Model file for the job. Use its own axes, mm. A direction names the side the tool comes from. Coordinates: 2 decimals unless noted, no trailing zeros. Write each loop counter-clockwise with the first axis right and the second up, starting at its lowest first coordinate (ties: lowest second). Pieces come first, ordered by that corner, then holes.
Q1. Band-saw the part on D-D, the plane y = -48.5. Write the cut outline in (x, z), plus the area to 3 significant figures.
Q2. Band-saw the part on C-C, the plane y = -26. Write the cut outline in (x, z).
Q3. Which spindle directions (+Z, -Z, +X, -X, +Y, -Y) get a long thin tool onto all of the face, cutting with end or side? Do faces 1 (the flat face through (18, 26.5, 17)), 2 (the flat face through (17.71, -15.74, 43.2)), 3 (the flat face through (-17.063, -2.368, 24.694)). Say none if no direction does.
Q4. Band-saw the part on A-A, the plane x = -51.5. Write the cut outline in (y, z).
Q5. Pin check, flat tips, straight feed: P1, Ø7, axis at x = -51.5, y = 48.5, coming from the +Z side; P2, Ø9.5, axis at y = -27.5, z = 33, coming from the -X side; P3, Ø5, axis at x = 7.5, z = 26.5, coming from the -Y side. Stop position of each tip, or through.
Q6. Band-saw the part on B-B, the plane y = 48.5. Write the cut outline in (x, z), plus the area to 3 significant figures.
Q7. Drill centre lines: probe 1 along Y at (x, z) = (-51.5, 17.25); probe 2 along Y at (x, z) = (51.5, 16.4); probe 3 along X at (y, z) = (48, 17). Where is each one in solid material? Low to high.
Q8. Pull direction Y, two halves, no side cores. Call faces 4 (the flat face through (-56.5, -1, 17)), 5 (the flat face through (-1, 53.5, 17)), 6 (the flat face through (-14.972, -17.284, 37.298)): released by +Y, released by -Y, zero draft, split by the parting line, or undercut.
from build123d import *

# Parameters (mm, degrees)
SKETCH1_W           = 113
SKETCH1_H           = 107
BOSS_EXTRUDE1_DEPTH = 20
SKETCH2_W           = 93
SKETCH2_H           = 87
CUT_EXTRUDE1_DEPTH  = 15
BOSS_EXTRUDE4_DEPTH = 20.5
SKETCH7_W           = 23
SKETCH7_H           = 10
CUT_EXTRUDE2_DEPTH  = 41
SKETCH10_R          = 3.727648652
SKETCH10_R_2        = 3.099940234
SKETCH10_R_3        = 3.503081025
SKETCH10_R_4        = 3.946186921
CUT_EXTRUDE3_DEPTH  = 94.259123843
SKETCH12_R          = 2
CUT_EXTRUDE5_DEPTH  = 10
CUT_EXTRUDE6_DEPTH  = 1.675
SKETCH15_W          = 118.362800564
SKETCH15_H          = 111.14113597
CUT_EXTRUDE7_DEPTH  = 86.907098164


with BuildPart() as part:
    # Sketch1 → Boss-Extrude1 (new body)
    with BuildSketch(Plane.XY):
        Rectangle(SKETCH1_W, SKETCH1_H)
    extrude(amount=BOSS_EXTRUDE1_DEPTH)

    # Sketch2 → Cut-Extrude1 (cut)
    with BuildSketch(Plane(origin=(0, 0, 0), x_dir=(-1, 0, 0), z_dir=(0, 0, -1))):
        Rectangle(SKETCH2_W, SKETCH2_H)
    extrude(amount=-CUT_EXTRUDE1_DEPTH, mode=Mode.SUBTRACT)

    # Sketch9 → Boss-Extrude4 (add, symmetric)
    with BuildSketch(Plane.ZY):
        Polygon((20, -53.5), (51.407822168, -16.069615096), (20, 10.284676901), align=None)
    extrude(amount=BOSS_EXTRUDE4_DEPTH, both=True)

    # Sketch7 → Cut-Extrude2 (cut)
    with BuildSketch(Plane(origin=(0, 0, 15), x_dir=(-1, 0, 0), z_dir=(0, 0, -1))):
        with Locations((-18, 31.5)):
            Rectangle(SKETCH7_W, SKETCH7_H)
        with Locations((14, 31.5)):
            Rectangle(SKETCH7_W, SKETCH7_H)
    extrude(amount=-CUT_EXTRUDE2_DEPTH, mode=Mode.SUBTRACT)

    # Sketch10 → Cut-Extrude3 (cut, through all)
    with BuildSketch(Plane(origin=(0, 0, 0), x_dir=(-1, 0, 0), z_dir=(0, 0, -1))):
        with Locations((-51.5, 48.5)):
            Circle(SKETCH10_R)
        with Locations((51.5, 48.5)):
            Circle(SKETCH10_R_2)
        with Locations((51.5, -48.5)):
            Circle(SKETCH10_R_3)
        with Locations((-51.5, -48.5)):
            Circle(SKETCH10_R_4)
    extrude(amount=-CUT_EXTRUDE3_DEPTH, mode=Mode.SUBTRACT)

    # Sketch12 → Cut-Extrude5 (cut)
    with BuildSketch(Plane(origin=(0, 15.883373682, 13.327732998), x_dir=(1, 0, 0), z_dir=(0, 0.7660444431189817, 0.6427876096865348))):
        with Locations(Location((-15, -19.710025981, 0), (0, 0, 270))):
            Circle(SKETCH12_R)
        with Locations(Location((15, -19.710025981, 0), (0, 0, 270))):
            Circle(SKETCH12_R)
        with Locations(Location((-14.999896364, -39.710025981, 0), (0, 0, 270))):
            Circle(SKETCH12_R)
        with Locations(Location((15, -39.710025981, 0), (0, 0, 270))):
            Circle(SKETCH12_R)
    extrude(amount=-CUT_EXTRUDE5_DEPTH, mode=Mode.SUBTRACT)

    # Sketch14 → Cut-Extrude6 (cut, symmetric)
    with BuildSketch(Plane(origin=(0, 12.053151466, 10.11379495), x_dir=(1, 0, 0), z_dir=(0, 0.7660444431189817, 0.6427876096865348))):
        with BuildLine():
            Line((-20.5, -16.210025981), (-20.5, -23.210025981))
            Line((-20.5, -23.210025981), (-15, -23.210025981))
            ThreePointArc((-15, -23.210025981), (-11.5, -19.710025981), (-15, -16.210025981))
            Line((-15, -16.210025981), (-20.5, -16.210025981))
        make_face()
        with BuildLine():
            Line((-20.5, -36.210025981), (-20.5, -43.210025981))
            Line((-20.5, -43.210025981), (-14.999896364, -43.210025981))
            ThreePointArc((-14.999896364, -43.210025981), (-11.499896364, -39.710025981), (-14.999896364, -36.210025981))
            Line((-14.999896364, -36.210025981), (-20.5, -36.210025981))
        make_face()
        with BuildLine():
            Line((20.5, -43.210025981), (20.5, -36.210025981))
            Line((20.5, -36.210025981), (15, -36.210025981))
            ThreePointArc((15, -36.210025981), (11.5, -39.710025981), (15, -43.210025981))
            Line((15, -43.210025981), (20.5, -43.210025981))
        make_face()
        with BuildLine():
            Line((20.5, -23.210025981), (20.5, -16.210025981))
            Line((20.5, -16.210025981), (15, -16.210025981))
            ThreePointArc((15, -16.210025981), (11.5, -19.710025981), (15, -23.210025981))
            Line((15, -23.210025981), (20.5, -23.210025981))
        make_face()
    extrude(amount=CUT_EXTRUDE6_DEPTH, both=True, mode=Mode.SUBTRACT)

    # Sketch15 → Cut-Extrude7 (cut, through all)
    with BuildSketch(Plane(origin=(0, 0, 15), x_dir=(-1, 0, 0), z_dir=(0, 0, -1))):
        Rectangle(SKETCH15_W, SKETCH15_H)
    extrude(amount=CUT_EXTRUDE7_DEPTH, mode=Mode.SUBTRACT)


solid = part.part
Answer sheet:
1. outline: (-56.5, 15) - (-55, 15) - (-55, 20) - (-56.5, 20) - close; (-48, 15) - (47.55, 15) - (47.55, 20) - (20.5, 20) - (20.5, 24.2) - (-20.5, 24.2) - (-20.5, 20) - (-48, 20) - close; (55.45, 15) - (56.5, 15) - (56.5, 20) - (55.45, 20) - close
1. area: 663 mm2
2. outline: (-56.5, 15) - (56.5, 15) - (56.5, 20) - (20.5, 20) - (20.5, 43.08) - (-20.5, 43.08) - (-20.5, 20) - (-56.5, 20) - close
3. face 1: +Z, -Z
3. face 2: +X
3. face 3: -X
4. outline: (-53.5, 15) - (-52, 15) - (-52, 20) - (-53.5, 20) - close; (-45, 15) - (45.4, 15) - (45.4, 20) - (-45, 20) - close; (51.6, 15) - (53.5, 15) - (53.5, 20) - (51.6, 20) - close
5. P1: stops at z = 20
5. P2: stops at x = -20.5
5. P3: stops at y = -48.73
6. outline: (-56.5, 15) - (-54.6, 15) - (-54.6, 20) - (-56.5, 20) - close; (-48.4, 15) - (47.77, 15) - (47.77, 20) - (-48.4, 20) - close; (55.23, 15) - (56.5, 15) - (56.5, 20) - (55.23, 20) - close
6. area: 497 mm2
7. probe 1: y = -53.5 to -52, -45 to 45.4, 51.6 to 53.5
7. probe 2: y = -53.5 to -52.45, -44.55 to 44.77, 52.23 to 53.5
7. probe 3: x = -56.5 to -54.56, -48.44 to 47.81, 55.19 to 56.5
8. face 4: zero draft
8. face 5: released by +Y
8. face 6: undercut
